The model under review builds one solid part; all positions refer to its coordinate system, in mm. Round coordinates to 2 decimals unless told otherwise and drop trailing zeros. Write each loop counter-clockwise with the first axis right and the second up, starting at its lowest first coordinate (ties: lowest second). Pieces come first, ordered by that corner, then holes. Notation, with made-up numbers: (42, -6) -> (93, -6) arc R20 ccw to (93, 1) -> close; hole circle Ø9 at (-8.5, 22.5). An arc over 180 degrees is marked (long way). Answer as a JSON object with one key per item and string values. Group by question number.
1) We need section B-B, the plane x = 37.5. Write out the cut boundary in (y, z), then the cut area to 3 significant figures.
2) Insertion check: pin 1 Ø1.5 at (x, y) = (64, 3.5) entering from -Z; pin 2 Ø1 at (y, z) = (3, -71.5) entering from +X; pin 3 Ø1.5 at (y, z) = (1.5, -38.5) entering from -X. Each pin has a flat end and moves straight along its axis. Give the tip position at first contact, or say it passes through.
3) We need section A-A, the plane y = 3.3. Write out the cut boundary in (x, z).
4) We need section C-C, the plane z = -52.5. Write out the cut boundary in (x, y), then the cut area to 3 significant figures.
5) To check wall thickness, follow probe 1 along X at (y, z) = (3.4, -85); probe 2 along Z at (x, y) = (31.5, 3.4); probe 3 along X at (y, z) = (2, -24.5). State the ranges of each line that lie inside material, in increasing order. Write a range as [from, to].
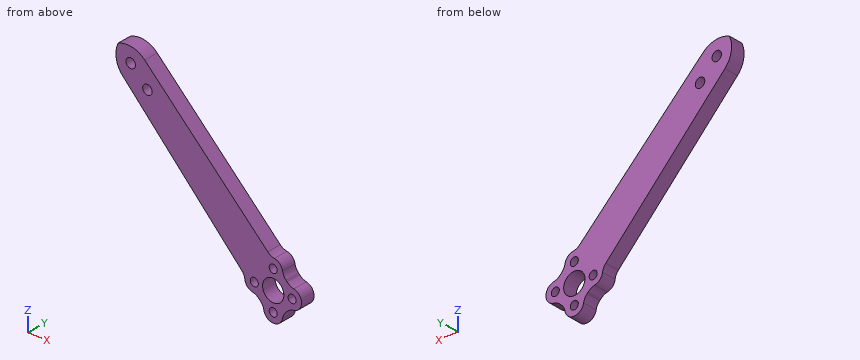
from build123d import *

# Parameters (mm, degrees)
SKETCH2_R               = 1.7
SKETCH2_R_2             = 4.5
BOSS_EXTRUDE1_DEPTH     = 6
FILLET1_R               = 10
CUT_EXTRUDE2_DEPTH      = 138.309868546
CUT_EXTRUDE2_DEPTH_BACK = 138.309868546
SKETCH7_R               = 2


with BuildPart() as part:
    # Sketch2 → Boss-Extrude1 (new body)
    with BuildSketch(Plane(origin=(0, 0, 0), x_dir=(1, 0, 0), z_dir=(0, 1, 0))):
        with BuildLine():
            Line((82.701229094, 71.670763572), (23.580603164, 14.468001358))
            Line((23.580603164, 14.468001358), (14.468001358, 23.580603164))
            Line((14.468001358, 23.580603164), (71.670763572, 82.701229094))
            ThreePointArc((71.670763572, 82.701229094), (72.579468699, 84.002771186), (73.034411761, 85.523555075))
            ThreePointArc((73.034411761, 85.523555075), (74.120868496, 87.776797037), (76.333333333, 88.944053189))
            ThreePointArc((76.333333333, 88.944053189), (77.868327334, 89.470595445), (79.153846154, 90.460996723))
            ThreePointArc((79.153846154, 90.460996723), (79.343145751, 90.656854249), (79.539003277, 90.846153846))
            ThreePointArc((79.539003277, 90.846153846), (80.529404555, 92.131672666), (81.055946811, 93.666666667))
            ThreePointArc((81.055946811, 93.666666667), (85, 97), (88.944053189, 93.666666667))
            ThreePointArc((88.944053189, 93.666666667), (89.470595445, 92.131672666), (90.460996723, 90.846153846))
            ThreePointArc((90.460996723, 90.846153846), (90.656854249, 90.656854249), (90.846153846, 90.460996723))
            ThreePointArc((90.846153846, 90.460996723), (92.131672666, 89.470595445), (93.666666667, 88.944053189))
            ThreePointArc((93.666666667, 88.944053189), (97, 85), (93.666666667, 81.055946811))
            ThreePointArc((93.666666667, 81.055946811), (92.131672666, 80.529404555), (90.846153846, 79.539003277))
            ThreePointArc((90.846153846, 79.539003277), (90.656854249, 79.343145751), (90.460996723, 79.153846154))
            ThreePointArc((90.460996723, 79.153846154), (89.470595445, 77.868327334), (88.944053189, 76.333333333))
            ThreePointArc((88.944053189, 76.333333333), (87.776797037, 74.120868496), (85.523555075, 73.034411761))
            ThreePointArc((85.523555075, 73.034411761), (84.002771186, 72.579468699), (82.701229094, 71.670763572))
        make_face()
        with Locations(Location((85, 93, 0), (0, 0, 270))):
            Circle(SKETCH2_R, mode=Mode.SUBTRACT)
        with Locations(Location((93, 85, 0), (0, 0, 270))):
            Circle(SKETCH2_R, mode=Mode.SUBTRACT)
        with Locations(Location((85, 77, 0), (0, 0, 270))):
            Circle(SKETCH2_R, mode=Mode.SUBTRACT)
        with Locations(Location((77, 85, 0), (0, 0, 270))):
            Circle(SKETCH2_R, mode=Mode.SUBTRACT)
        with Locations(Location((85, 85, 0), (0, 0, 270))):
            Circle(SKETCH2_R_2, mode=Mode.SUBTRACT)
    extrude(amount=BOSS_EXTRUDE1_DEPTH)

    # Fillet1
    # the kernel refuses this fillet: 10 mm, written as the material it takes off along each edge
    with BuildSketch(Plane(origin=(23.580603164, -24.591214075, -14.468001358), x_dir=(0.71866742198992, 0, -0.6953539649490483), z_dir=(0, 1, 0)), Plane(origin=(14.468001358, -24.591214075, -23.580603164), x_dir=(0.7071067811865477, 0, 0.7071067811865475), z_dir=(0, 1, 0))) as fillet1_piece_1:
        with BuildLine():
            CenterArc((FILLET1_R * 0.983648563013, FILLET1_R), FILLET1_R, 180.944569645, 89.055430355)
            Line((-FILLET1_R * 0.0162155484343, FILLET1_R * 0.983514896433), (0, 0))
            Line((0, 0), (FILLET1_R * 0.983648563013, 0))
        make_face()
    extrude(amount=55.182428151, mode=Mode.SUBTRACT)

    # Sketch7 → Cut-Extrude2 (cut, two sides: drawn at the far end of the back side and taken through both)
    with BuildSketch(Plane(origin=(0, 0, 0), x_dir=(1, 0, 0), z_dir=(0, 1, 0)).offset(-CUT_EXTRUDE2_DEPTH_BACK)):
        with Locations(Location((24.748737342, 24.748737342, 0), (0, 0, 270))):
            Circle(SKETCH7_R)
        with Locations(Location((31.819805153, 31.819805153, 0), (0, 0, 270))):
            Circle(SKETCH7_R)
    extrude(amount=CUT_EXTRUDE2_DEPTH + CUT_EXTRUDE2_DEPTH_BACK, mode=Mode.SUBTRACT)


solid = part.part
Here are the results:
{
 "1": {"outline": "(0, -47.38) -> (6, -47.38) -> (6, -27.94) -> (0, -27.94) -> close", "area": "117 mm^2"},
 "2": {"pin 1": "stops at z = -75.55", "pin 2": "stops at x = 83.08", "pin 3": "stops at x = 28.18"},
 "3": {"outline": "(19.44, -19.44) arc R10 ccw to (21.31, -30.65) -> (71.67, -82.7) arc R5 cw to (73.03, -85.52) arc R4 ccw to (76.33, -88.94) arc R5 cw to (79.15, -90.46) arc R8 ccw to (79.54, -90.85) arc R5 cw to (81.06, -93.67) arc R4 ccw to (88.94, -93.67) arc R5 cw to (90.46, -90.85) arc R8 ccw to (90.85, -90.46) arc R5 cw to (93.67, -88.94) arc R4 ccw to (93.67, -81.06) arc R5 cw to (90.85, -79.54) arc R8 ccw to (90.46, -79.15) arc R5 cw to (88.94, -76.33) arc R4 ccw to (85.52, -73.03) arc R5 cw to (82.7, -71.67) -> (30.65, -21.31) arc R10 ccw to start; hole circle Ø4 at (24.75, -24.75); hole circle Ø4 at (31.82, -31.82); hole circle Ø3.4 at (77, -85); hole circle Ø9 at (85, -85); hole circle Ø3.4 at (85, -93); hole circle Ø3.4 at (85, -77); hole circle Ø3.4 at (93, -85)"},
 "4": {"outline": "(42.45, 0) -> (62.89, 0) -> (62.89, 6) -> (42.45, 6) -> close", "area": "123 mm^2"},
 "5": {"probe 1": "x = [72.94, 75.3], [78.7, 80.5], [89.5, 91.3], [94.7, 97]", "probe 2": "z = [-41.18, -33.79], [-29.85, -22.13]", "probe 3": "x = [18.53, 22.76], [26.73, 33.95]"}
}
